Input: part model. Units: mm. Frame: model coordinates. Face numbers are marked on the shaded views. A direction names the side the tool comes from. Coordinates: 2 decimals unless noted, no trailing zeros. Write each loop counter-clockwise with the first axis right and the second up, starting at its lowest first coordinate (ties: lowest second). Pieces come first, ordered by that corner, then holes. Notation, with made-up numbers: M 48.25,-34.5 L 83.25,-34.5 A7 ccw 83.25,-28.5 Z; hole C -23.75,54.5 d10. An arc over 180 degrees is marked long. Use one line per item in the form item = value.
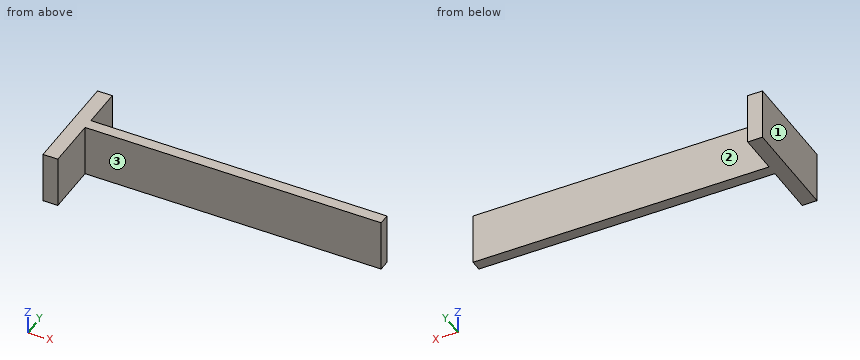
Autodesk Inventor part; units mm, degrees
ref_plane "Work Plane2" through (0, -16, -7) normal (0, -1, 0) x (1, 0, 0)
ref_plane "YZ Plane" through (0, 0, 0) normal (1, 0, 0) x (0, 1, 0)
ref_plane "XZ Plane" through (0, 0, 0) normal (0, 1, 0) x (-1, 0, 0)
ref_plane "Work Plane1" through (0, 0, 0) normal (0, 0, 1) x (1, 0, 0)
sketch "Sketch1" plane through (0, 0, 0) normal (0, 0, 1) x (1, 0, 0)
  line L0 (0, 0) -> (0, -15.5)
  line L1 (0, -15.5) -> (30, -15.5)
  line L2 (30, -0.5) -> (30, -15.5)
  line L3 (0, -0.5) -> (30, -0.5)
  line L4 (30, -0.5) -> (-10, -0.5)
  line L5 (-10, -0.5) -> (-10, 1.5)
  line L6 (-10, 1.5) -> (30, 1.5)
  line L7 (30, 1.5) -> (30, -0.5)
  point P0 (0, -0.5)
  dimension "d0" = 40
  dimension "d1" = 2
extrude "Extrusion1" add sketch "Sketch1" against normal up to surface (7 mm away) contours L4 L5 L6 L7 L3
ref_plane "Work Plane2" through (0, -16, -7) normal (0, -1, 0) x (1, 0, 0)
move faces "Move1" translate (0, -0.5, 0) faces at (16.6667, 1.5, -2.3333)
sketch "Sketch3" plane through (-10, -0.5, 0) normal (0, -1, 0) x (1, 0, 0)
  line L0 (40, 0) -> (0, 0)
  line L1 (0, 0) -> (-2, 0)
  line L2 (-2, 0) -> (-2, -7)
  line L3 (-2, -7) -> (0, -7)
  line L4 (0, -7) -> (0, 0)
  point P0 (10, 0)
  dimension "d19" = 2
extrude "Extrusion3" add sketch "Sketch3" along normal blind 7 and the other way blind 7
properties part number "fence"
(1) Section query C-C on x = 16.5. Return the cut outline in (y, z).
Computed:
outline = M -0.5,-7 L 1,-7 L 1,0 L -0.5,0 Z
(2) Section query B-B on y = -3. Return the cut outline in (x, z), plus the area to 3 significant figures.
Computed:
outline = M -12,-7 L -10,-7 L -10,0 L -12,0 Z
area = 14.0 mm^2
(3) Line query: probe 1 along Y at (x, z) = (4, -2.5); probe 2 along X at (y, z) = (-1.75, -2.75). Output: solid intervals per line, ascending.
Computed:
probe_1 = -0.5 to 1
probe_2 = -12 to -10
(4) First-contact query: pin 1 Ø2 at (x, z) = (19, -5.5) entering from -Y; pin 2 Ø3 at (y, z) = (3.5, -2.5) entering from +X; pin 3 Ø3.5 at (x, z) = (1, -5) entering from +Y. Flat tips, straight axial feed; report the tip coordinate or a pass-through.
Computed:
pin_1 = -0.5
pin_2 = -10
pin_3 = 1
(5) Section query A-A on z = -5. Return the cut outline in (x, y), plus the area to 3 significant figures.
Computed:
outline = M -12,-7.5 L -10,-7.5 L -10,-0.5 L 30,-0.5 L 30,1 L -10,1 L -10,6.5 L -12,6.5 Z
area = 88.0 mm^2
(6) Set-up query: the marked faces 1, 2 and 3. Return all of +Z, -Z, +X, -X, +Y, -Y with unobstructed straight access to the full face (end or side cutting, diameter ignored); none if empty.
Computed:
face_1 = +Z, -Z, -X, +Y, -Y
face_2 = +Z, -Z, +X, +Y
face_3 = +Z, -Z, +X, -Y
